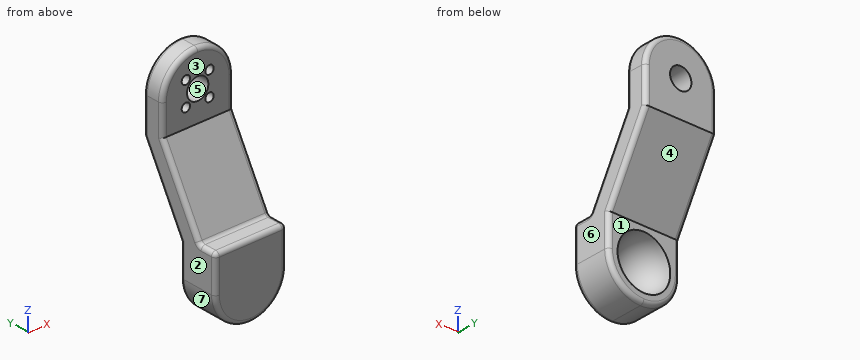
from build123d import *

# Parameters (mm, degrees)
PROFILEEXTRUDE_THIN1_DEPTH          = 34
DOMEPADEXTENSIONSKETCH1_W           = 34
DOMEPADEXTENSIONSKETCH1_H           = 34.639067238
DOMEPADEXTENSIONBOSS_EXTRUDE1_DEPTH = 8.8
FILLET1_R                           = 17
FILLET2_R                           = 17
FLANGENUTHOLESKETCH4_R              = 5.1
FLANGENUTHOLECUT_EXTRUDE5_DEPTH     = 114.638162666
DOMEINDENTSKETCH6_R                 = 12.6
DOMEINDENTCUT_EXTRUDE8_DEPTH        = 0.1
DOME2_FACE_RADIUS                   = 12.6
DOME2_HEIGHT                        = 12.5
FILLET3_R                           = 17
FILLET4_R                           = 17
BOTTOMBOUNDARYFILLET5_R             = 2
FLANGENUTHOLESSKETCH2_R             = 2
FLANGENUTHOLESCUT_EXTRUDE1_DEPTH    = 4
FILLET6_R                           = 2


with BuildPart() as part:
    # ProfileSketch1 → ProfileExtrude-Thin1 (new body)
    with BuildSketch(Plane(origin=(0, 0, 0), x_dir=(0, 0, -1), z_dir=(1, 0, 0))):
        Polygon((0, 0), (34, 0), (69.253108664, -20), (101.253108664, -20), (101.253108664, -30), (66.614041426, -30), (31.360932762, -10), (0, -10), align=None)
    extrude(amount=PROFILEEXTRUDE_THIN1_DEPTH)

    # DomePadExtensionSketch1 → DomePadExtensionBoss-Extrude1 (add)
    with BuildSketch(Plane.XZ.offset(30)):
        with Locations((17, -83.933575045)):
            Rectangle(DOMEPADEXTENSIONSKETCH1_W, DOMEPADEXTENSIONSKETCH1_H)
    extrude(amount=DOMEPADEXTENSIONBOSS_EXTRUDE1_DEPTH)

    # Fillet1
    fillet1_edges = [part.edges().sort_by_distance(p)[0] for p in [
        (34, -5, 0),
    ]]
    fillet(fillet1_edges, radius=FILLET1_R)

    # Fillet2
    fillet2_edges = [part.edges().sort_by_distance(p)[0] for p in [
        (0, -5, 0),
    ]]
    fillet(fillet2_edges, radius=FILLET2_R - 0.0001)  # a hair under: the kernel refuses the full size

    # FlangeNutHoleSketch4 → FlangeNutHoleCut-Extrude5 (cut, through all)
    with BuildSketch(Plane(origin=(0, 0, 0), x_dir=(1, 0, 0), z_dir=(0, 1, 0))):
        with Locations(Location((17, 17, 0), (0, 0, 270))):
            Circle(FLANGENUTHOLESKETCH4_R)
    extrude(amount=-FLANGENUTHOLECUT_EXTRUDE5_DEPTH, mode=Mode.SUBTRACT)

    # DomeIndentSketch6 → DomeIndentCut-Extrude8 (cut)
    with BuildSketch(Plane(origin=(0, -20, 0), x_dir=(1, 0, 0), z_dir=(0, 1, 0))):
        with Locations(Location((17, 84.253108664, 0), (0, 0, 270))):
            Circle(DOMEINDENTSKETCH6_R)
    extrude(amount=-DOMEINDENTCUT_EXTRUDE8_DEPTH, mode=Mode.SUBTRACT)

    # Dome2: a dome of height H over a round flat face of radius A is a cap of a sphere of radius (A * A + H * H) / (2 * H)
    dome2_r = (DOME2_FACE_RADIUS * DOME2_FACE_RADIUS + DOME2_HEIGHT * DOME2_HEIGHT) / (2 * DOME2_HEIGHT)
    dome2_base = Plane((17, -20.1, -84.253108664), z_dir=(0, -1, 0))
    with Locations(dome2_base.offset(DOME2_HEIGHT - dome2_r)):
        dome2_ball = Sphere(dome2_r, mode=Mode.PRIVATE)
    add(split(dome2_ball, bisect_by=dome2_base, keep=Keep.TOP, mode=Mode.PRIVATE), mode=Mode.SUBTRACT)

    # Fillet3
    fillet3_edges = [part.edges().sort_by_distance(p)[0] for p in [
        (34, -29.4, -101.253108664),
    ]]
    fillet(fillet3_edges, radius=FILLET3_R)

    # Fillet4
    fillet4_edges = [part.edges().sort_by_distance(p)[0] for p in [
        (0, -29.4, -101.253108664),
    ]]
    fillet(fillet4_edges, radius=FILLET4_R - 0.0001)  # a hair under: the kernel refuses the full size

    # BottomBoundaryFillet5
    bottomboundaryfillet5_edges = [part.edges().sort_by_distance(p)[0] for p in [
        (17, -30, -66.614041426),
        (0, -34.4, -66.614041426),
        (34, -34.4, -66.614041426),
        (0, -38.8, -75.433625045),
        (17, -38.8, -66.614041426),
        (34, -20, -48.987487094),
        (34, -10, -24.180466381),
        (29.02081528, -10, -4.97918472),
        (0, -10, -24.180416381),
        (4.979155431, -10, -4.979155431),
        (34, -38.8, -75.433575045),
        (29.02081528, -38.8, -96.273923944),
        (4.979155431, -38.8, -96.273953234),
        (0, -20, -48.987487094),
    ]]
    fillet(bottomboundaryfillet5_edges, radius=BOTTOMBOUNDARYFILLET5_R)

    # FlangeNutHolesSketch2 → FlangeNutHolesCut-Extrude1 (cut)
    with BuildSketch(Plane.XZ.offset(10)):
        with Locations(Location((11.343145751, -11.343145751, 0), (0, 0, 270))):
            Circle(FLANGENUTHOLESSKETCH2_R)
        with Locations(Location((22.656854249, -11.343145751, 0), (0, 0, 270))):
            Circle(FLANGENUTHOLESSKETCH2_R)
        with Locations(Location((22.656854249, -22.656854249, 0), (0, 0, 270))):
            Circle(FLANGENUTHOLESSKETCH2_R)
        with Locations(Location((11.343145751, -22.656854249, 0), (0, 0, 270))):
            Circle(FLANGENUTHOLESSKETCH2_R)
    extrude(amount=-FLANGENUTHOLESCUT_EXTRUDE1_DEPTH, mode=Mode.SUBTRACT)

    # Fillet6
    fillet6_edges = [part.edges().sort_by_distance(p)[0] for p in [
        (34, -20, -76.753108664),
        (34, -10, -51.626554332),
        (34, 0, -25.5),
        (29.02081528, 0, -4.97918472),
        (0, 0, -25.49995),
        (4.979155431, 0, -4.979155431),
        (29.02081528, -20, -96.273923944),
        (4.979155431, -20, -96.273953234),
        (0, -10, -51.626554332),
        (0, -20, -76.753158664),
    ]]
    fillet(fillet6_edges, radius=FILLET6_R)


solid = part.part
Work out the finished part from the listing and answer in its coordinate system (mm). Face numbers are marked on the shaded views. A direction names the side the tool comes from. Give positions to 0.01 mm unless a question says otherwise; leave off trailing zeros. Answer in a Markdown table with one row per item. Add a question column.
Q1. Consider line 1 along Y through (x, z) = (10, -13.5); line 2 along Y through (x, z) = (10, -73); line 3 along Z through (x, y) = (22, -20.5). Determine where each line is inside the solid, lowest interval first.
Q2. Each of these flat-tipped pins is pushed along its axis until it touches: P1, Ø15, axis at x = 17, z = -91, coming from the +Y side; P2, Ø13.5, axis at x = 17, z = -17, coming from the -Y side; P3, Ø5, axis at x = 20.5, z = -42.5, coming from the +Y side. Where does it stop, or does it pass through?
Q3. A tool of negligible diameter and unlimited length cuts with its end or side. For the marked faces 1, 2 and 3, from which of +Z, -Z, +X, -X, +Y, -Y can it reach the whole face along a straight path? Write none if from no direction.
Q4. Determine the mould class of the marked faces 4, 5, 6 and 7 for opening direction X: released by +X, released by -X, zero draft, split by the parting line, or undercut.
Solution:
| question | item | result |
|---|---|---|
| 1 | line 1 | y = -10 to 0 |
| 1 | line 2 | y = -38.8 to -20 |
| 1 | line 3 | z = -99.79 to -95.81, -72.7 to -49.87 |
| 2 | P1 | stops at y = -20 |
| 2 | P2 | stops at y = -10 |
| 2 | P3 | stops at y = -3.4 |
| 3 | face 1 | -Z, +X, -X, +Y |
| 3 | face 2 | +Z, -Z, -X, +Y, -Y |
| 3 | face 3 | +Z, +X, -X, -Y |
| 4 | face 4 | zero draft |
| 4 | face 5 | undercut |
| 4 | face 6 | released by +X |
| 4 | face 7 | released by -X |
